from build123d import *

# Parameters (mm, degrees)
BOSS_EXTRUDE1_DEPTH             = 3.175
F_6_CLEARANCE_HOLE1_D           = 4.3053
F_4_CLEARANCE_HOLE1_D           = 3.4544
F_6_CLEARANCE_HOLE2_D           = 4.3053
F_9_64_0_14063_DIAMETER_HOLE1_D = 3.572002
F_3_8_0_375_DIAMETER_HOLE1_D    = 9.525
F_1_2_0_5_DIAMETER_HOLE1_D      = 12.7


with BuildPart() as part:
    # Sketch1 → Boss-Extrude1 (new body)
    with BuildSketch(Plane.XY):
        Polygon((112.268, 0), (0, 0), (0, -148.336), (112.268, -138.684), align=None)
    extrude(amount=-BOSS_EXTRUDE1_DEPTH)

    # #6 Clearance Hole1 (through all)
    with Locations(Plane.XY):
        with Locations((6.731, -133.35), (107.3785, -128.5875), (107.3785, -66.675), (4.8895, -76.2)):
            Hole(F_6_CLEARANCE_HOLE1_D / 2)

    # #4 Clearance Hole1 (through all)
    with Locations(Plane.XY):
        with Locations((18.644469576, -70.03220158), (57.60279842, -62.459469576), (65.175530424, -101.41779842), (26.21720158, -108.990530424), (65.891864398, -135.837535562), (88.720535562, -134.641135602), (87.524135602, -111.812464438), (64.695464438, -113.008864398)):
            Hole(F_4_CLEARANCE_HOLE1_D / 2)

    # #6 Clearance Hole2 (through all)
    with Locations(Plane.XY):
        with Locations((36.322, -16.51), (85.6615, -47.625)):
            Hole(F_6_CLEARANCE_HOLE2_D / 2)

    # 9/64 (0.14063) Diameter Hole1 (through all)
    with Locations(Plane.XY):
        with Locations((27.051, -22.352)):
            Hole(F_9_64_0_14063_DIAMETER_HOLE1_D / 2)

    # 3/8 (0.375) Diameter Hole1 (through all)
    with Locations(Plane.XY):
        with Locations((76.2, -25.4)):
            Hole(F_3_8_0_375_DIAMETER_HOLE1_D / 2)

    # 1/2 (0.5) Diameter Hole1 (through all)
    with Locations(Plane.XY):
        with Locations((17.526, -22.352)):
            Hole(F_1_2_0_5_DIAMETER_HOLE1_D / 2)


solid = part.part
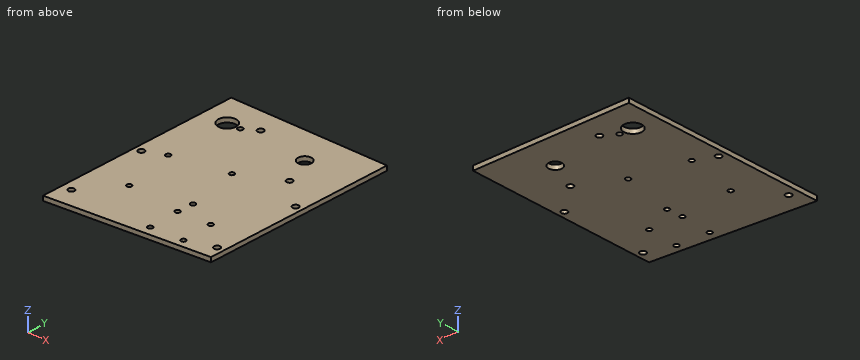
Input: part model. Units: mm. Frame: model coordinates. Coordinates: 2 decimals unless noted, no trailing zeros. Loops run counter-clockwise (first coordinate to the right, second up) from the corner with the lowest first, then second, coordinate; pieces in that order, holes last. Notation, with made-up numbers: (-11.75, -1.5) -> (23.25, -1.5) arc R13 cw to (23.25, 16.5) -> close; hole circle Ø5 at (47.25, 58.5). An arc over 180 degrees is marked (long way). Write each question's results on one line, items separated by ' | '. Start each with the question number.
Q1. Section A-A, the plane y = -76.2. Return the cut outline in (x, z) (3 decimals).
Q2. Ray query, line 1 (X direction, y = -47.5, z = -1.2); line 2 (X direction, y = -74.5, z = -1.8); line 3 (X direction, y = -27.5, z = -1.15). Return the intervals inside material, ascending. Write a range as from..to.
Q3. Section B-B, the plane x = 76.2. Return the cut outline in (y, z) (1 decimal).
Q4. Pin query (flat end, axial travel): pin 1 (1 mm diameter, centred on x = 60, z = -1.5, fed in from -Y). Return the tip coordinate at first contact, or that it passes through.
Q5. Section C-C, the plane z = -1.5. State how many separate pieces and enclosed holes the cut face has, plus the area to 3 significant figures.
Found:
1) outline: (0, -3.175) -> (2.737, -3.175) -> (2.737, 0) -> (0, 0) -> close; (7.042, -3.175) -> (112.268, -3.175) -> (112.268, 0) -> (7.042, 0) -> close
2) line 1: 0..83.51, 87.81..112.27 | line 2: 0..3.57, 6.21..112.27 | line 3: 0..13.81, 21.24..71.93, 80.47..112.27
3) outline: (-141.8, -3.2) -> (-30.2, -3.2) -> (-30.2, 0) -> (-141.8, 0) -> close; (-20.6, -3.2) -> (0, -3.2) -> (0, 0) -> (-20.6, 0) -> close
4) pin 1: y = -143.22
5) separate pieces: 1 | enclosed holes: 17 | area: 15,700 mm2
